from build123d import *

# Parameters (mm, degrees)
SKETCH1_R                = 17.45
SKETCH1_R_2              = 12.45
BOSS_EXTRUDE1_DEPTH      = 8
BOSS_EXTRUDE1_DEPTH_BACK = 25
SKETCH2_R                = 20.25
SKETCH2_R_2              = 12.45
BOSS_EXTRUDE2_DEPTH      = 40
SKETCH3_R                = 17.5
SKETCH3_R_2              = 12.45
CUT_EXTRUDE1_DEPTH       = 221
SKETCH4_W                = 78.3000253
SKETCH4_H                = 101.772836534
CUT_EXTRUDE2_DEPTH       = 221
CUT_EXTRUDE2_DEPTH_BACK  = 221
SKETCH5_R                = 1
CUT_EXTRUDE3_DEPTH       = 221
CUT_EXTRUDE4_START       = -19
SKETCH6_R                = 2.5
CUT_EXTRUDE4_DEPTH       = 221
CIRPATTERN1_COUNT        = 3


with BuildPart() as part:
    # Sketch1 → Boss-Extrude1 (new body, two sides)
    with BuildSketch(Plane(origin=(0, 0, 0), x_dir=(1, 0, 0), z_dir=(0, 1, 0))) as boss_extrude1_sk:
        Circle(SKETCH1_R)
        Circle(SKETCH1_R_2, mode=Mode.SUBTRACT)
    extrude(amount=BOSS_EXTRUDE1_DEPTH)
    extrude(boss_extrude1_sk.sketch, amount=-BOSS_EXTRUDE1_DEPTH_BACK)

    # Sketch2 → Boss-Extrude2 (add)
    with BuildSketch(Plane(origin=(0, 8, 0), x_dir=(1, 0, 0), z_dir=(0, 1, 0))):
        Circle(SKETCH2_R)
        Circle(SKETCH2_R_2, mode=Mode.SUBTRACT)
    extrude(amount=BOSS_EXTRUDE2_DEPTH)

    # Sketch3 → Cut-Extrude1 (cut)
    with BuildSketch(Plane(origin=(0, 48, 0), x_dir=(1, 0, 0), z_dir=(0, 1, 0))):
        Circle(SKETCH3_R)
        Circle(SKETCH3_R_2, mode=Mode.SUBTRACT)
    extrude(amount=-CUT_EXTRUDE1_DEPTH, mode=Mode.SUBTRACT)

    # Sketch4 → Cut-Extrude2 (cut, two sides)
    with BuildSketch(Plane(origin=(0, 0, 0), x_dir=(0, 0, -1), z_dir=(1, 0, 0))) as cut_extrude2_sk:
        with Locations((-0.109307072, 64.886418267)):
            Rectangle(SKETCH4_W, SKETCH4_H)
    extrude(amount=CUT_EXTRUDE2_DEPTH, mode=Mode.SUBTRACT)
    extrude(cut_extrude2_sk.sketch, amount=-CUT_EXTRUDE2_DEPTH_BACK, mode=Mode.SUBTRACT)

    # Sketch5 → Cut-Extrude3 (cut)
    with BuildSketch(Plane.XY):
        with Locations((0, 11)):
            Circle(SKETCH5_R)
    cut_extrude3 = extrude(amount=-CUT_EXTRUDE3_DEPTH, mode=Mode.SUBTRACT)

    # Sketch6 → Cut-Extrude4 (cut)
    with BuildSketch(Plane.XY.offset(CUT_EXTRUDE4_START)):
        with Locations((0, 11)):
            Circle(SKETCH6_R)
    cut_extrude4 = extrude(amount=-CUT_EXTRUDE4_DEPTH, mode=Mode.SUBTRACT)

    # CirPattern1: Cut-Extrude3, Cut-Extrude4 ×3 about axis
    cirpattern1_axis = Axis((0, 0, 0), (0, 1, 0))
    for i in range(1, CIRPATTERN1_COUNT):
        add(cut_extrude3.rotate(cirpattern1_axis, i * 360 / CIRPATTERN1_COUNT), mode=Mode.SUBTRACT)
        add(cut_extrude4.rotate(cirpattern1_axis, i * 360 / CIRPATTERN1_COUNT), mode=Mode.SUBTRACT)


solid = part.part
Check sheet for the modelled part. Datum: model origin and axes. Units: mm. A direction names the side the tool comes from. Round coordinates to 2 decimals unless told otherwise and drop trailing zeros. Loops run counter-clockwise (first coordinate to the right, second up) from the corner with the lowest first, then second, coordinate; pieces in that order, holes last. Notation, with made-up numbers: (-12, 73.5) -> (9, 73.5) arc R16 cw to (9, 80.5) -> close; hole circle Ø8 at (-20, 78.5). An arc over 180 degrees is marked (long way). Put each result on its own line as item: value. Start each with the question number.
1. Section check D-D (x = -10.5). Enter the section's corners in (y, z).
2. Access from +Z, -Z, +X, -X, +Y, -Y to the whole of each face (thin tool, end or side, straight path). Record for faces 1 (the face through (2.31, 10.04, -19.62)), 2 (the face through (-13.887, 11.042, 10.648)), 3 (the face through (16.194, 9.924, 9.951)).
3. Section check A-A (z = 0). Enter the section's corners in (x, y).
4. Scan lines: probe 1 along Y at (x, z) = (0, -20); probe 2 along X at (y, z) = (12.75, 0); probe 3 along Y at (x, z) = (0, -18.05). Record each from-to range of solid material in increasing order.
5. Section check B-B (x = 0). Enter the section's corners in (y, z), plus the area to 4 significant figures.
6. Gauge pin test, flat ends, axial feed: pin 1 (1.6 mm diameter, centred on x = 0, y = 11, fed in from -Z); pin 2 (2.5 mm diameter, centred on x = 1, y = 10.5, fed in from -Z); pin 3 (1.5 mm diameter, centred on x = 14.5, y = 11.5, fed in from +Z). Record the tip position at first contact, or that the pin passes through.
7. Draft check along X on faces 4 (the face through (0, 10, -18)), 5 (the face through (6, 14, 17)), 6 (the face through (11, 11, -17)). Enter one of: +X half, -X half, draft (parallel to the pull), parting line (faces both ways), or undercut.
8. Section check C-C (y = 11.5). Enter the section's corners in (x, z), plus the area to 3 significant figures.
Findings:
1. outline: (8, -17.32) -> (14, -17.32) -> (14, -14) -> (8, -14) -> close; (8, 14) -> (14, 14) -> (14, 17.32) -> (8, 17.32) -> close
2. face 1: -Z
2. face 2: +Y, -Y
2. face 3: none
3. outline: (-20.25, 8) -> (-17.5, 8) -> (-17.5, 14) -> (-20.25, 14) -> close; (17.5, 8) -> (20.25, 8) -> (20.25, 14) -> (17.5, 14) -> close
4. probe 1: y = 8 to 8.5, 13.5 to 14
4. probe 2: x = -20.25 to -17.5, 17.5 to 20.25
4. probe 3: y = 8 to 10, 12 to 14
5. outline: (8, -20.25) -> (8.5, -20.25) -> (8.5, -19) -> (10, -19) -> (10, -17.5) -> (8, -17.5) -> close; (8, 17.5) -> (14, 17.5) -> (14, 20.25) -> (8, 20.25) -> close; (12, -19) -> (13.5, -19) -> (13.5, -20.25) -> (14, -20.25) -> (14, -17.5) -> (12, -17.5) -> close
5. area: 23.75 mm^2
6. pin 1: stops at z = 17.48
6. pin 2: stops at z = -19
6. pin 3: stops at z = 14.87
7. face 4: undercut
7. face 5: draft
7. face 6: parting line
8. outline: (-18.63, 7.93) arc R20.25 ccw to (-2.45, -20.1) -> (-2.45, -19) -> (-0.87, -19) -> (-0.87, -17.48) arc R17.5 cw to (-15.57, 7.99) -> (-16.89, 8.75) -> (-17.68, 7.38) -> close; (-16.18, 12.17) -> (-15.23, 11.62) -> (-16.02, 10.25) -> (-14.7, 9.49) arc R17.5 cw to (14.7, 9.49) -> (16.02, 10.25) -> (15.23, 11.62) -> (16.18, 12.17) arc R20.25 ccw to start; (0.87, -19) -> (2.45, -19) -> (2.45, -20.1) arc R20.25 ccw to (18.63, 7.93) -> (17.68, 7.38) -> (16.89, 8.75) -> (15.57, 7.99) arc R17.5 cw to (0.87, -17.48) -> close
8. area: 301 mm^2
